The model under review builds one solid part; all positions refer to its coordinate system, in mm. Face numbers are marked on the shaded views. A direction names the side the tool comes from. Coordinates: 2 decimals unless noted, no trailing zeros. Order: outer loops, then holes, each group sorted by start corner. A loop starts at its lowest first (then second) coordinate and runs counter-clockwise, first axis right, second up.
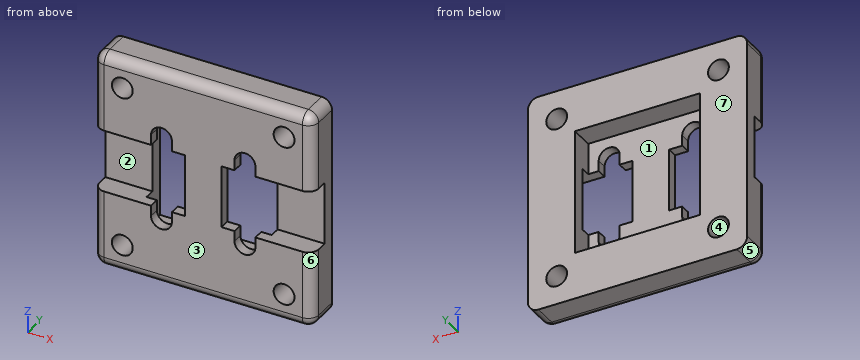
Autodesk Inventor part; units mm, degrees
ref_plane "Work Plane4" through (25, 0, 21) normal (1, 0, 0) x (0, 0, -1)
ref_plane "YZ Plane" through (0, 0, 0) normal (1, 0, 0) x (0, 1, 0)
ref_plane "XZ Plane" through (0, 0, 0) normal (0, 1, 0) x (-1, 0, 0)
sketch "Sketch1" plane through (0, 0, 0) normal (0, 1, 0) x (-1, 0, 0)
  line L0 (21, 21) -> (-21, 21)
  line L1 (-21, 21) -> (-21, -21)
  line L2 (-21, -21) -> (21, -21)
  line L3 (21, -21) -> (21, 21)
  line L4 (21, 21) -> (-21, -21) construction
  line L5 (-21, 21) -> (21, -21) construction
  point P0 (0, 0)
  dimension "d0" = 42
  dimension "d1" = 42
extrude "Extrusion1" add sketch "Sketch1" along normal blind 6.5
sketch "Sketch2" plane through (0, 6.5, 0) normal (0, 1, 0) x (1, 0, 0)
  line L0 (-12, -12) -> (12, -12)
  line L1 (12, -12) -> (12, 12)
  line L2 (12, 12) -> (-12, 12)
  line L3 (-12, 12) -> (-12, -12)
  line L4 (-12, -12) -> (12, 12) construction
  line L5 (12, -12) -> (-12, 12) construction
  point P0 (0, 0)
  dimension "d4" = 24
  dimension "d5" = 24
extrude "Extrusion2" cut sketch "Sketch2" against normal blind 4.5
sketch "Sketch3" plane through (0, 2, 0) normal (0, 1, 0) x (1, 0, 0)
  line L0 (-10.5, -6) -> (-3.5, -6)
  line L1 (-3.5, -6) -> (-3.5, 6)
  line L2 (-3.5, 6) -> (-10.5, 6)
  line L3 (-10.5, 6) -> (-10.5, -6)
  line L4 (-10.5, -6) -> (-3.5, 6) construction
  line L5 (-3.5, -6) -> (-10.5, 6) construction
  line L6 (-12, -12) -> (-12, 12)
  line L7 (3.5, -6) -> (10.5, -6)
  line L8 (10.5, -6) -> (10.5, 6)
  line L9 (10.5, 6) -> (3.5, 6)
  line L10 (3.5, 6) -> (3.5, -6)
  line L11 (3.5, -6) -> (10.5, 6) construction
  line L12 (10.5, -6) -> (3.5, 6) construction
  line L13 (12, 12) -> (12, -12)
  point P0 (0, 0)
  point P1 (-7, 0)
  point P2 (-7, 0)
  point P3 (7, 0)
  point P4 (7, 0)
  dimension "d8" = 7
  dimension "d9" = 12
  dimension "d10" = 1.5
  dimension "d11" = 7
  dimension "d12" = 1.5
  dimension "d13" = 12
extrude "Extrusion3" cut sketch "Sketch3" against normal blind 3.5
sketch "Sketch4" plane through (0, 2, 0) normal (0, 1, 0) x (1, 0, 0)
  line L0 (-12, -12) -> (-12, 12)
  line L1 (12, -12) -> (-12, -12)
  point P0 (0, 0)
  point P1 (-8, -8)
  point P2 (-8, 8)
  point P3 (8, 8)
  point P4 (8, -8)
  dimension "d16" = 16
  dimension "d17" = 16
  dimension "d18" = 4
  dimension "d19" = 4
hole "Hole1" at (-8, 2, 8) at (-8, 2, -8) at (8, 2, -8) at (8, 2, 8) direction (0, -1, 0) diameter 4 end through all
sketch "Sketch5" plane through (0, 6.5, 0) normal (0, 1, 0) x (1, 0, 0)
  line L0 (-21, -21) -> (21, -21)
  line L1 (-21, 21) -> (-21, -21)
  point P0 (0, 0)
  point P1 (-15.5, -15.5)
  point P2 (-15.5, 15.5)
  point P3 (15.5, 15.5)
  point P4 (15.5, -15.5)
  dimension "d27" = 31
  dimension "d28" = 31
  dimension "d29" = 5.5
  dimension "d30" = 5.5
hole "Hole2" at (-15.5, 6.5, 15.5) at (-15.5, 6.5, -15.5) at (15.5, 6.5, -15.5) at (15.5, 6.5, 15.5) direction (0, -1, 0) diameter 4 end through all
sketch "Sketch8" plane through (0, 0, 0) normal (0, -1, 0) x (1, 0, 0)
  line L0 (-21, -21) -> (-21, 21)
  line L1 (-21, 21) -> (-25, 21)
  line L2 (-25, 21) -> (-25, -21)
  line L3 (-25, -21) -> (-21, -21)
  line L4 (-21, -21) -> (-21, 21)
  line L5 (21, -21) -> (-21, -21)
  point P0 (0, 0)
  point P1 (25, -21)
  dimension "d48" = 4
extrude "Extrusion6" add sketch "Sketch8" against normal blind 46.5
sketch "Sketch9" plane through (-25, 0, -21) normal (-1, 0, 0) x (0, 0, 1)
  point P0 (21, 0)
ref_plane "Work Plane4" through (25, 0, 21) normal (1, 0, 0) x (0, 0, -1)
sketch "Sketch10" plane through (25, 0, 21) normal (1, 0, 0) x (0, 0, -1)
  line L0 (27, 2) -> (31, 2)
  line L1 (27, 2) -> (15, 2)
  line L2 (11, 2) -> (15, 2)
  line L3 (15, 2) -> (27, 2)
  line L4 (27, 2) -> (31, 2)
  line L5 (27, 2) -> (15, 2)
  line L6 (11, 2) -> (15, 2)
  line L7 (15, 2) -> (27, 2)
  line L8 (33, 2) -> (9, 2)
  line L9 (9, 2) -> (33, 2)
  line L10 (27, 2) -> (15, 2)
  line L11 (27, 2) -> (27, 0)
  line L12 (15, 2) -> (27, 2)
  line L13 (15, 2) -> (15, 0)
  line L14 (27, 0) -> (15, 0)
  point P0 (21, 0)
extrude "Extrusion7" cut sketch "Sketch10" against normal blind 15
sketch "Sketch11" plane through (-25, 0, -21) normal (-1, 0, 0) x (0, 0, 1)
  line L0 (27, 2) -> (27, 0)
  line L1 (15, 2) -> (27, 2)
  line L2 (15, 2) -> (15, 0)
  line L3 (27, 0) -> (15, 0)
  point P0 (21, 0)
extrude "Extrusion8" cut sketch "Sketch11" against normal blind 15
sketch "Sketch12" plane through (-25, 0, 6) normal (-1, 0, 0) x (0, 0, 1)
  line L0 (-27, 0) -> (-27, 46.5)
  point P0 (-6, 0)
  point P1 (-21, 41.5)
  point P2 (9, 41.5)
  point P3 (9, 11.5)
  point P4 (-21, 11.5)
  point P5 (-27, 5.5)
  dimension "d55" = 30
  dimension "d56" = 30
  dimension "d57" = 6
  dimension "d92" = 6
hole "Hole3" at (-25, 11.5, -15) at (-25, 11.5, 15) at (-25, 41.5, -15) at (-25, 41.5, 15) direction (1, 0, 0) diameter 3.5 depth 8 tip angle 118
sketch "Sketch13" plane through (-25, 0, 6) normal (-1, 0, 0) x (0, 0, 1)
  circle A0 centre (-21, 41.5) radius 1.75
  circle A1 centre (-21, 11.5) radius 1.75
  circle A2 centre (9, 11.5) radius 1.75
  circle A3 centre (9, 41.5) radius 1.75
  line L0 (0, 2) -> (0, 0)
  line L1 (15, 0) -> (0, 0)
  line L2 (15, 0) -> (15, 46.5)
  line L3 (-27, 46.5) -> (15, 46.5)
  line L4 (-27, 0) -> (-27, 46.5)
  line L5 (-12, 0) -> (-12, 2)
  line L6 (-12, 2) -> (0, 2)
  circle A4 centre (-21, 41.5) radius 3.25
  circle A5 centre (9, 41.5) radius 3.25
  circle A6 centre (9, 11.5) radius 3.25
  circle A7 centre (-21, 11.5) radius 3.25
  line L7 (-12, 0) -> (-27, 0)
  point P0 (-6, 0)
  dimension "d65" = 1.5
  dimension "d66" = 1.5
  dimension "d67" = 1.5
  dimension "d68" = 1.5
extrude "Extrusion9" add sketch "Sketch13" along normal blind 2 contours A4 | A5 | A6 | A7
fillet "Fillet2" radius 5 2 edges at (-23, 46.5, -21) (-23, 46.5, 21)
fillet "Fillet3" radius 1 4 edges at (-25, 11.5, 11.75) (-25, 41.5, 11.75) (-25, 41.5, -18.25) (-25, 11.5, -18.25)
sketch "Sketch16" plane through (-25, 2, -6) normal (0, -1, 0) x (1, 0, 0)
  line L0 (13, 12) -> (13, 0)
  line L1 (0, 12) -> (13, 12)
  line L2 (0, 0) -> (0, 12)
  line L3 (0, 0) -> (13, 0)
  line L4 (37, 0) -> (37, 12)
  line L5 (50, 0) -> (37, 0)
  line L6 (50, 12) -> (50, 0)
  line L7 (50, 12) -> (37, 12)
  point P0 (25, 6)
extrude "Extrusion11" cut sketch "Sketch16" against normal blind 2
sketch "Sketch17" plane through (-21, 6.5, 21) normal (1, 0, 0) x (0, 0, -1)
  arc A0 (5, 40) -> (0, 35) centre (5, 35) ccw
  line L0 (0, 0) -> (0, 35)
  line L1 (42, 0) -> (0, 0)
  line L2 (42, 0) -> (42, 35)
  arc A1 (42, 35) -> (37, 40) centre (37, 35) ccw
  line L3 (5, 40) -> (37, 40)
  circle A2 centre (36, 35) radius 1.75
  circle A3 centre (36, 5) radius 1.75
  circle A4 centre (6, 5) radius 1.75
  circle A5 centre (6, 35) radius 1.75
  point P0 (21, -6.5)
extrude "Extrusion12" cut sketch "Sketch17" against normal blind 0.8
sketch "Sketch19" plane through (-25, 0, 6) normal (-1, 0, 0) x (0, 0, 1)
  line L0 (6.5, 18.2831) -> (-6, 11.0662)
  line L1 (-6, 11.0662) -> (-18.5, 18.2831)
  line L2 (-18.5, 18.2831) -> (-18.5, 32.7169)
  line L3 (-18.5, 32.7169) -> (-6, 39.9338)
  line L4 (-6, 39.9338) -> (6.5, 32.7169)
  line L5 (6.5, 32.7169) -> (6.5, 18.2831)
  line L6 (-27, 0) -> (-27, 41.5)
  line L7 (-22, 46.5) -> (10, 46.5)
  point P0 (-6, 0)
  point P1 (-6, 25.5)
  dimension "d104" = 25
  dimension "d105" = 21
  dimension "d106" = 21
extrude "Extrusion14" cut sketch "Sketch19" against normal through all
fillet "Fillet4" radius 2 18 edges at (-23.4, 32.7169, -12.5) (-23.4, 39.9338, 0) (-23.4, 18.2831, -12.5) (-23.4, 11.0662, 0) (-23.4, 18.2831, 12.5) (-23.4, 32.7169, 12.5) (-25, 4, 0) (-25, 45.0355, 19.5355) (-25, 46.5, 0) (-25, 45.0355, -19.5355) (-25, 20.75, -21) (-25, 20.75, 21) (21, 0, -13.5) (21, 0, 13.5) (-25, 0, -13.5) (-25, 0, 13.5) (-2, 0, -21) (-2, 0, 21)
sketch "Sketch20" plane through (-21.8, 6.5, 21) normal (1, 0, 0) x (0, 0, -1)
  circle A0 centre (6, 35) radius 2.75
  circle A1 centre (6, 35) radius 1.75
  point P0 (21, -6.5)
  dimension "d110" = 5.5
extrude "Extrusion15" cut sketch "Sketch20" against normal blind 3
pattern_linear "Rectangular Pattern2" count 2 spacing 30 along (0, 0, -1) count 2 spacing 30 along (0, -1, 0) of "Extrusion15"
sketch "Sketch21" plane through (0, 0, 0) normal (0, -1, 0) x (1, 0, 0)
  circle A0 centre (8, 8) radius 2
  circle A1 centre (8, -8) radius 2
  circle A2 centre (-8, -8) radius 2
  circle A3 centre (-8, 8) radius 2
  circle A4 centre (-8, 8) radius 2
  line L0 (-10, 8) -> (-6, 8)
  line L1 (-6, 8) -> (-6, -8)
  line L2 (-6, -8) -> (-10, -8)
  line L3 (-10, -8) -> (-10, 8)
  line L4 (6, 8) -> (10, 8)
  line L5 (10, 8) -> (10, -8)
  line L6 (10, -8) -> (6, -8)
  line L7 (6, -8) -> (6, 8)
  point P0 (0, 0)
  point P1 (8, 6)
  point P2 (8, -6)
  point P3 (-8, -6)
  point P4 (-8, 6)
  point P5 (10, 8)
  point P6 (-6, 8)
extrude "Extrusion16" cut sketch "Sketch21" against normal blind 3 contours L5 A1 L7 A0 | A2 L3 A3 L1
sketch "Sketch22" plane through (-21.8, 6.5, 21) normal (1, 0, 0) x (0, 0, -1)
  circle A0 centre (36, 5) radius 2.75
  circle A1 centre (6, 5) radius 2.75
  circle A2 centre (36, 35) radius 2.75
  circle A3 centre (6, 35) radius 2.75
  line L0 (22, 32.8564) -> (32.5, 26.7942)
  arc A4 (33.5, 25.0622) -> (32.5, 26.7942) centre (31.5, 25.0622) ccw
  line L1 (33.5, 25.0622) -> (33.5, 12.9378)
  arc A5 (32.5, 11.2058) -> (33.5, 12.9378) centre (31.5, 12.9378) ccw
  line L2 (32.5, 11.2058) -> (22, 5.1436)
  arc A6 (20, 5.1436) -> (22, 5.1436) centre (21, 6.8756) ccw
  line L3 (20, 5.1436) -> (9.5, 11.2058)
  arc A7 (8.5, 12.9378) -> (9.5, 11.2058) centre (10.5, 12.9378) ccw
  line L4 (8.5, 12.9378) -> (8.5, 25.0622)
  arc A8 (9.5, 26.7942) -> (8.5, 25.0622) centre (10.5, 25.0622) ccw
  line L5 (9.5, 26.7942) -> (20, 32.8564)
  arc A9 (22, 32.8564) -> (20, 32.8564) centre (21, 31.1244) ccw
  arc A10 (42, 35) -> (37, 40) centre (37, 35) ccw
  line L6 (5, 40) -> (37, 40)
  arc A11 (5, 40) -> (0, 35) centre (5, 35) ccw
  line L7 (0, 0) -> (0, 35)
  line L8 (42, 0) -> (0, 0)
  line L9 (42, 35) -> (42, 0)
  circle A12 centre (36, 35) radius 1.75
  circle A13 centre (36, 5) radius 1.75
  circle A14 centre (6, 5) radius 1.75
  circle A15 centre (6, 35) radius 1.75
  point P0 (21, -6.5)
extrude "Extrusion17" cut sketch "Sketch22" against normal blind 10 contours A0 | A1 | A2 | A3 | L9 L8 L7 A11 L6 A10 | A12 | A13 | A14 | A15
fillet "Fillet5" radius 2 4 edges at (20.4142, 0.5858, 20.4142) (21, 4.25, 21) (20.4142, 0.5858, -20.4142) (21, 4.25, -21)
sketch "Sketch23" plane through (0, 6.5, 0) normal (0, 1, 0) x (1, 0, 0)
  circle A0 centre (15.5, 15.5) radius 2
  circle A1 centre (-15.5, -15.5) radius 2
  circle A2 centre (-15.5, 15.5) radius 2
  circle A3 centre (15.5, -15.5) radius 2
  line L0 (-12, 12) -> (12, 12)
  line L1 (12, 12) -> (12, -12)
  line L2 (12, -12) -> (-12, -12)
  line L3 (-12, -12) -> (-12, 12)
  arc A4 (21, 19) -> (19, 21) centre (19, 19) ccw
  line L4 (19, 21) -> (-23, 21)
  arc A5 (-23, 21) -> (-25, 19) centre (-23, 19) ccw
  line L5 (-25, -19) -> (-25, 19)
  arc A6 (-25, -19) -> (-23, -21) centre (-23, -19) ccw
  line L6 (19, -21) -> (-23, -21)
  arc A7 (19, -21) -> (21, -19) centre (19, -19) ccw
  line L7 (21, -19) -> (21, 19)
  line L8 (0, 0) -> (21, 0)
  line L9 (0, 0) -> (-21, 0)
  line L10 (-21, 0) -> (-21, 21)
  line L11 (-21, 0) -> (-21, -21)
  dimension "d124" = 21
  dimension "d125" = 21
extrude "Extrusion18" cut sketch "Sketch23" against normal blind 10 contours L11 L6 A6 L5 A5 L4 L10
fillet "Fillet6" radius 2 5 edges at (-21, 0.5858, -20.4142) (-21, 0, -12.5) (-21, 4.25, -21) (-21, 0.5858, 20.4142) (-21, 4.25, 21)
properties part number "Soporte base PCBs"
(1) We need section D-D, the plane y = 5. Write out the cut boundary in (x, z).
A:
outline: (-21, -19) arc R2 ccw to (-19, -21) - (19, -21) arc R2 ccw to (21, -19) - (21, 19) arc R2 ccw to (19, 21) - (-19, 21) arc R2 ccw to (-21, 19) - close; hole circle Ø4 at (-15.5, -15.5); hole circle Ø4 at (-15.5, 15.5); hole (-12, -12) - (12, -12) - (12, 12) - (-12, 12) - close; hole circle Ø4 at (15.5, -15.5); hole circle Ø4 at (15.5, 15.5)
(2) For pin 1 Ø7 at (x, z) = (-14.5, -1.5) entering from -Y; pin 2 Ø1.5 at (x, y) = (-15.5, 1) entering from -Z; pin 3 Ø0.6 at (x, y) = (-4, 1) entering from -Z, all flat-tipped, find the tip position at first contact; note any pin that passes through.
A:
pin 1: stops at y = 4
pin 2: stops at z = -20.98
pin 3: stops at z = -20.87
(3) Machinability: for the marked faces 1, 2 and 3, which of the approach directions +Z, -Z, +X, -X, +Y, -Y give a long, thin tool a straight path to every point of the face, cutting with its end or side? Answer none if there is none.
A:
face 1: +Y
face 2: +X, -X, -Y
face 3: +Z, -Z, +X, -X, -Y
(4) Draft analysis for pull direction X (two halves, no side actions). For the marked faces 4, 5, 6 and 7, state which applies: released by +X, released by -X, zero draft, split by the parting line, or undercut.
A:
face 4: undercut
face 5: released by -X
face 6: released by +X
face 7: zero draft
(5) We need section B-B, the plane z = -5.5. Write out the cut boundary in (x, y).
A:
outline: (-21, 4) - (-12, 4) - (-12, 6.5) - (-21, 6.5) - close; (-3.5, 0) - (3.5, 0) - (3.5, 2) - (-3.5, 2) - close; (12, 4) - (21, 4) - (21, 6.5) - (12, 6.5) - close
(6) We need section A-A, the plane x = -5. Write out the cut boundary in (y, z), and give its area (3 significant figures).
A:
outline: (0, -19) arc R2 ccw to (2, -21) - (6.5, -21) - (6.5, -12) - (2, -12) - (2, -6) - (0, -6) - close; (0, 6) - (2, 6) - (2, 12) - (6.5, 12) - (6.5, 21) - (2, 21) arc R2 ccw to (0, 19) - close
area: 139 mm2
(7) We need section C-C, the plane x = -15.5. Write out the cut boundary in (y, z).
A:
outline: (0, -19) arc R2 ccw to (2, -21) - (6.5, -21) - (6.5, -17.5) - (0, -17.5) - close; (0, -13.5) - (6.5, -13.5) - (6.5, 13.5) - (0, 13.5) - (0, 6) - (4, 6) - (4, -6) - (0, -6) - close; (0, 17.5) - (6.5, 17.5) - (6.5, 21) - (2, 21) arc R2 ccw to (0, 19) - close
(8) Wall thickness on probe 1 along X at (y, z) = (4.75, -15.5); probe 2 along Z at (x, y) = (-3.5, 4.5): over which ranges is each line inside the solid? List them lowest first.
A:
probe 1: x = -21 to -17.5, -13.5 to 13.5, 17.5 to 21
probe 2: z = -21 to -12, 12 to 21
